Geometry check sheet. Reference: the model listing, model coordinates, mm. A direction names the side the tool comes from. Coordinates: 2 decimals unless noted, no trailing zeros. Write each loop counter-clockwise with the first axis right and the second up, starting at its lowest first coordinate (ties: lowest second). Pieces come first, ordered by that corner, then holes. Notation, with made-up numbers: (-17, 5) -> (3, 5) arc R19 ccw to (3, 10) -> close; hole circle Ø2 at (-23, 83). An arc over 180 degrees is marked (long way). Use a Markdown table: item, result.
Autodesk Fusion 360 part; units mm, degrees
sketch "Esquisse1" plane through (0, 0, 0) normal (0, 0, 1) x (1, 0, 0)
  line L0 (0, 0) -> (30, 0)
  line L1 (30, 0) -> (30, 5)
  line L2 (30, 5) -> (10, 5)
  line L3 (10, 5) -> (10, 8)
  line L4 (10, 8) -> (30, 8)
  line L5 (30, 8) -> (30, 13)
  line L6 (30, 13) -> (10, 13)
  line L7 (10, 13) -> (0, 23)
  line L8 (0, 23) -> (-11.5, 11.5)
  line L9 (-11.5, 11.5) -> (0, 0)
  dimension "d2" = 3
  dimension "d3" = 5
  dimension "d4" = 20
  dimension "d5" = 30
  dimension "d6" = 20
  dimension "d7" = 15
  dimension "d8" = 135
  dimension "d22" = 13
extrude "Extrusion1" add sketch "Esquisse1" along normal blind 125 makes body 1
chamfer "Chanfrein2" distance 2 angle 25 1 edges at (30, 8, 62.5) measured on face at (16.6667, 8, 41.6667) on bodies 1
sketch "Esquisse2" plane through (0, 0, 0) normal (0, -1, 0) x (1, 0, 0)
  line L0 (0, 0) -> (30, 0)
  line L1 (30, 0) -> (30, 125)
  line L2 (30, 125) -> (0, 125)
  line L3 (0, 125) -> (0, 0)
  circle A0 centre (20, 12.85) radius 1.7
  line L4 (18.3546, 15.7) -> (16.7091, 12.85)
  line L5 (16.7091, 12.85) -> (18.3546, 10)
  line L6 (18.3546, 10) -> (21.6454, 10)
  line L7 (21.6454, 10) -> (23.2909, 12.85)
  line L8 (23.2909, 12.85) -> (21.6454, 15.7)
  line L9 (21.6454, 15.7) -> (18.3546, 15.7)
  line L10 (0, 0) -> (30, 0)
  point P0 (20, 12.85)
  point P1 (-10, 0)
  point P2 (-30, 125)
  dimension "d11" = 3.4
  dimension "d12" = 2.85
  dimension "d15" = 10
  dimension "d16" = 10
extrude "Extrusion2" cut sketch "Esquisse2" against normal blind 13 contours A0 bodies 1
chamfer "Chanfrein1" distance 2 angle 45 1 edges at (18.415, 0, 13.4647) on bodies 1
sketch "Esquisse3" plane through (0, 13, 0) normal (0, 1, 0) x (-1, 0, 0)
  circle A0 centre (-20, 12.85) radius 1.7
  line L0 (-30, 0) -> (-10, 0)
  line L1 (-10, 0) -> (-10, 125)
  line L2 (-10, 125) -> (-30, 125)
  line L3 (-30, 125) -> (-30, 0)
  line L4 (-18.3546, 15.7) -> (-21.6454, 15.7)
  line L5 (-21.6454, 15.7) -> (-23.2909, 12.85)
  line L6 (-23.2909, 12.85) -> (-21.6454, 10)
  line L7 (-21.6454, 10) -> (-18.3546, 10)
  line L8 (-18.3546, 10) -> (-16.7091, 12.85)
  line L9 (-16.7091, 12.85) -> (-18.3546, 15.7)
  point P0 (-20, 12.85)
  dimension "d23" = 2.85
extrude "Extrusion4" cut sketch "Esquisse3" against normal blind 3 contours L4 L5 L6 L7 L8 L9 bodies 1
ref_plane "Plan de construction2" through (-5.75, 17.25, 62.5) normal (-0.7071, 0.7071, 0) x (-0.7071, -0.7071, 0)
mirror "Symétrie miroir1" about plane through (-5.75, 17.25, 62.5) normal (-0.7071, 0.7071, 0) of bodies 1 merged
sketch "Esquisse4" plane through (0, 0, 0) normal (0, 0, 1) x (1, 0, 0)
  line L0 (10, 13) -> (-10, 33) construction
  line L1 (-6.2132, 8) -> (-6.2132, 16.7868) construction
  line L2 (-6.2132, 16.7868) -> (-15, 16.7868) construction
  line L3 (-6.2132, 16.7868) -> (0, 23) construction
  line L4 (29.8, 8) -> (8.2, 8) construction
  line L5 (-15, 52.8) -> (-15, 31.2) construction
  circle A0 centre (-6.2132, 16.7868) radius 2.5
  point P0 (-15, 8)
  dimension "d32" = 5
  dimension "d33" = 8.7868
extrude "Extrusion5" cut sketch "Esquisse4" along normal blind 35 bodies 1
ref_plane "Plan de construction3" through (3.5, 26.5, 125) normal (0, 0, 1) x (1, 0, 0)
mirror "Symétrie miroir2" about plane through (3.5, 26.5, 125) normal (0, 0, 1) of bodies 1 merged
sketch "Esquisse5" plane through (0, 0, 0) normal (0, 0, -1) x (1, 0, 0)
  line L0 (30, -8.9326) -> (28, -8)
  line L1 (28, -8) -> (10, -8)
  line L2 (10, -8) -> (10, -5)
  line L3 (10, -5) -> (30, -5)
  line L4 (30, -5) -> (30, 0)
  line L5 (30, 0) -> (0, 0)
  line L6 (0, 0) -> (-23, -23)
  line L7 (-23, -23) -> (-23, -53)
  line L8 (-23, -53) -> (-18, -53)
  line L9 (-18, -53) -> (-18, -33)
  line L10 (-18, -33) -> (-15, -33)
  line L11 (-15, -33) -> (-15, -51)
  line L12 (-15, -51) -> (-14.0674, -53)
  line L13 (-14.0674, -53) -> (-10, -53)
  line L14 (-10, -53) -> (-10, -33)
  line L15 (-10, -33) -> (10, -13)
  line L16 (10, -13) -> (30, -13)
  line L17 (30, -13) -> (30, -8.9326)
  line L18 (-15, -8) -> (185, -8)
  line L19 (185, -8) -> (185, -208)
  line L20 (185, -208) -> (-15, -208)
  line L21 (-15, -208) -> (-15, -8)
  circle A0 centre (-6.2132, -16.7868) radius 2.5
  dimension "d39" = 200
  dimension "d40" = 200
extrude "Extrusion6" cut sketch "Esquisse5" against normal blind 7 contours L0 L1 L6 L11 L12 L13 L14 L15 L16 L17 L18 L21 | L0 L12 L13 L14 L15 L16 L17 L18 L19 L20 L21 | A0 bodies 1
copy_body "Corps->Comp1" bodies 1 removing the originals makes body 2 in component "Component"
component "Component" placed x (1, 0, 0) y (0, 1, 0) z (0, 0, 1) at (0, 0, 0)
equation "d4 = d6 + 0 mm"
equation "d5 = d4 + 10 mm"
equation "d9 = ( 250 / 2 ) * 1 mm"
equation "d13 = -( 2 * d3 + d2 )"
equation "d15 = d6 / 2"
equation "d23 = d12"
equation "d27 = -d3 + 2 mm"
Item 1: Section check A-A on z = 123.5. Record the boundary of the cut face in (x, y).
Answer block:
| item | result |
|---|---|
| outline | (-23, 23) -> (0, 0) -> (30, 0) -> (30, 5) -> (10, 5) -> (10, 8) -> (28, 8) -> (30, 8.93) -> (30, 13) -> (10, 13) -> (-10, 33) -> (-10, 53) -> (-14.07, 53) -> (-15, 51) -> (-15, 33) -> (-18, 33) -> (-18, 53) -> (-23, 53) -> close |
Item 2: Mould release check, pull along Z, two halves, no side actions. Record for faces 4 (the flat face through (15, 0, 123)), 5 (the flat face through (-6, 17, 35)), 6 (the conical face through (19.604, 1.875, 235.368)): +Z half, -Z half, draft (parallel to the pull), parting line (faces both ways), or undercut.
Answer block:
| item | result |
|---|---|
| face 4 | draft |
| face 5 | -Z half |
| face 6 | undercut |
Item 3: Depth check by flat-ended pin: P1, Ø6.5, axis at y = 43.5, z = 236, coming from the +X side; P2, Ø22, axis at x = 17, z = 91.5, coming from the +Y side; P3, Ø4, axis at y = 43, z = 12.85, coming from the -X side; P4, Ø5, axis at x = 5.5, z = 126, coming from the -Y side. Enter the tip coordinate at first touch or a pass-through.
Answer block:
| item | result |
|---|---|
| P1 | stops at x = -10 |
| P2 | stops at y = 17 |
| P3 | stops at x = -21.3 |
| P4 | stops at y = 0 |
Item 4: Thickness scan on L1, parallel to Z at x = -13.7, y = 43; L2, parallel to Z at x = -19.4, y = 43; L3, parallel to X at y = 42, z = 186. Record the ranges inside material, lowest first. Write a range as [from, to].
Answer block:
| item | result |
|---|---|
| L1 | z = [7, 11.15], [14.55, 235.45], [238.85, 250] |
| L2 | z = [0, 11.15], [14.55, 235.45], [238.85, 250] |
| L3 | x = [-23, -18], [-15, -10] |
Item 5: Tool access check on faces 1 (the flat face through (20, 13, 127)), 2 (the flat face through (-13, 44.4, 11.6)), 3 (the cylindrical face through (-8.2, 15.27, 232.74)). Record the directions out of +Z, -Z, +X, -X, +Y, -Y that give a thin tool (end or side, any length) a straight path to the whole face; none if there is none.
Answer block:
| item | result |
|---|---|
| face 1 | +Z, -Z, +X, +Y |
| face 2 | +X |
| face 3 | +Z |
